Build history of the part. All positions in model axes, mm. A direction names the side the tool comes from. Give positions to 0.01 mm unless a question says otherwise; leave off trailing zeros. Write each loop counter-clockwise with the first axis right and the second up, starting at its lowest first coordinate (ties: lowest second). Pieces come first, ordered by that corner, then holes.
from build123d import *

# Parameters (mm, degrees)
CHAMFER1_SIZE      = 0.381
SKETCH2_R          = 2.667
CUT_EXTRUDE1_DEPTH = 6.35
SKETCH3_R          = 0.79375
CUT_EXTRUDE2_DEPTH = 23.030279682


with BuildPart() as part:
    # Sketch1 → Revolve1 (revolve)
    with BuildSketch(Plane.XY, mode=Mode.PRIVATE) as revolve1_sk:
        Polygon((0, 21.082), (0.79375, 21.082), (1.7526, 17.78), (1.7526, 15.24), (2.3622, 15.24), (2.3622, 8.89), (4.5212, 8.89), (4.5212, 0), (0, 0), align=None)
    revolve(revolve1_sk.sketch.rotate(Axis((0, 0, 0), (0, 1, 0)), 90), axis=Axis((0, 0, 0), (0, 1, 0)))

    # Chamfer1
    chamfer1_edges = [part.edges().sort_by_distance(p)[0] for p in [
        (0, 0, 4.5212),
        (0, 8.89, 4.5212),
    ]]
    chamfer(chamfer1_edges, length=CHAMFER1_SIZE)

    # Sketch2 → Cut-Extrude1 (cut)
    with BuildSketch(Plane.XZ):
        with Locations(Location((0, 0, 0), (0, 0, 270))):
            Circle(SKETCH2_R)
    extrude(amount=-CUT_EXTRUDE1_DEPTH, mode=Mode.SUBTRACT)

    # Sketch3 → Cut-Extrude2 (cut, through all)
    with BuildSketch(Plane(origin=(0, 21.082, 0), x_dir=(1, 0, 0), z_dir=(0, 1, 0))):
        with Locations(Location((0, 0, 0), (0, 0, 270))):
            Circle(SKETCH3_R)
    extrude(amount=-CUT_EXTRUDE2_DEPTH, mode=Mode.SUBTRACT)


solid = part.part
(1) 3-axis set-ups, long thin cutter, end or side, ignore diameter. For faces 4 (the face through (-1.99, 12.02, -1.27)), 5 (the face through (-1.62, 3.13, 2.12)), 6 (the face through (3, 0, 0)): which of +Z, -Z, +X, -X, +Y, -Y reach the whole face in a straight line?
(2) Mould opens along Z. For faces 1 (the face through (2, 8.89, 2)), 2 (the face through (4.414, 4.388, 0.98)), 3 (the face through (-0.48, 13.82, -0.63)) say: +Z half, -Z half, draft (parallel to the pull), parting line (faces both ways), or undercut.
(3) Saw through at D-D, the plane y = 18.5. List the corners of the cut face in (x, z), plus the area to 3 significant figures.
(4) Drop flat-ended pins along their axis: pin 1 (2.5 mm diameter, centred on x = -0.5, z = -0.5, fed in from +Y); pin 2 (1.6 mm diameter, centred on x = 0.5, z = 0.5, fed in from -Y); pin 3 (2 mm diameter, centred on x = 0.5, z = 3, fed in from +Y); pin 4 (3 mm diameter, centred on y = 9.5, z = -2.5, fed in from -X). Give the stop position or say it passes through.
(5) Saw through at C-C, the plane y = 16. List the corners of the cut face in (x, z).
(6) Saw through at A-A, the plane x = 0. List the corners of the cut face in (y, z), plus the area to 4 significant figures.
(7) Saw through at B-B, the plane z = 0. List the corners of the cut face in (x, y).
(8) Probe line 1 (X direction, y = 16, z = 0); line 2 (X direction, y = 1.25, z = 0); line 3 (Y direction, x = 0.5, z = -3.5). List the from-to ranges inside material, lowest first.
Computed values:
1. face 4: +Y
1. face 5: -Y
1. face 6: +Z, -Z, +X, -X, -Y
2. face 1: draft
2. face 2: parting line
2. face 3: undercut
3. outline: circle Ø3.09 at (0, 0); hole circle Ø1.59 at (0, 0)
3. area: 5.51 mm2
4. pin 1: stops at y = 21.08
4. pin 2: stops at y = 6.35
4. pin 3: stops at y = 15.24
4. pin 4: stops at x = -4.31
5. outline: circle Ø3.51 at (0, 0); hole circle Ø1.59 at (0, 0)
6. outline: (0, -4.14) - (0.38, -4.52) - (8.51, -4.52) - (8.89, -4.14) - (8.89, -2.36) - (15.24, -2.36) - (15.24, -1.75) - (17.78, -1.75) - (21.08, -0.79) - (6.35, -0.79) - (6.35, -2.67) - (0, -2.67) - close; (0, 2.67) - (6.35, 2.67) - (6.35, 0.79) - (21.08, 0.79) - (17.78, 1.75) - (15.24, 1.75) - (15.24, 2.36) - (8.89, 2.36) - (8.89, 4.14) - (8.51, 4.52) - (0.38, 4.52) - (0, 4.14) - close
6. area: 70.15 mm2
7. outline: (-4.52, 0.38) - (-4.14, 0) - (-2.67, 0) - (-2.67, 6.35) - (-0.79, 6.35) - (-0.79, 21.08) - (-1.75, 17.78) - (-1.75, 15.24) - (-2.36, 15.24) - (-2.36, 8.89) - (-4.14, 8.89) - (-4.52, 8.51) - close; (0.79, 6.35) - (2.67, 6.35) - (2.67, 0) - (4.14, 0) - (4.52, 0.38) - (4.52, 8.51) - (4.14, 8.89) - (2.36, 8.89) - (2.36, 15.24) - (1.75, 15.24) - (1.75, 17.78) - (0.79, 21.08) - close
8. line 1: x = -1.75 to -0.79, 0.79 to 1.75
8. line 2: x = -4.52 to -2.67, 2.67 to 4.52
8. line 3: y = 0 to 8.89
